Can you work these out from the model? Positions are in its coordinate system, mm. A direction names the side the tool comes from. Round coordinates to 2 decimals unless told otherwise and drop trailing zeros. Loops run counter-clockwise (first coordinate to the right, second up) from the corner with the lowest first, then second, coordinate; pieces in that order, holes last.
```python
from build123d import *

# Parameters (mm, degrees)
BOSS_EXTRUDE1_DEPTH = 9.525
SKETCH2_R           = 1.905
CUT_EXTRUDE1_DEPTH  = 9.525
SKETCH3_R           = 2.286
CUT_EXTRUDE2_DEPTH  = 78.455641076


with BuildPart() as part:
    # Sketch1 → Boss-Extrude1 (new body)
    with BuildSketch(Plane(origin=(0, 0, 0), x_dir=(0, 0, -1), z_dir=(1, 0, 0))):
        Polygon((0, 0), (-25.4, 0), (25.4, 72.549918742), (25.4, 12.7), (0, 12.7), align=None)
    extrude(amount=BOSS_EXTRUDE1_DEPTH)

    # Sketch2 → Cut-Extrude1 (cut)
    with BuildSketch(Plane.XZ.offset(-12.7)):
        with Locations(Location((4.7625, -19.05, 0), (0, 0, 270))):
            Circle(SKETCH2_R)
        with Locations(Location((4.7625, -6.35, 0), (0, 0, 270))):
            Circle(SKETCH2_R)
    extrude(amount=-CUT_EXTRUDE1_DEPTH, mode=Mode.SUBTRACT)

    # Sketch3 → Cut-Extrude2 (cut, through all)
    with BuildSketch(Plane(origin=(9.525, 0, 0), x_dir=(0, 0, -1), z_dir=(1, 0, 0))):
        with Locations((-6.35, 16.135332376)):
            Circle(SKETCH3_R)
        with Locations((15.503262225, 47.345025264)):
            Circle(SKETCH3_R)
    extrude(amount=-CUT_EXTRUDE2_DEPTH, mode=Mode.SUBTRACT)


solid = part.part
```
(1) Which directions (+Z, -Z, +X, -X, +Y, -Y) give clear straight access to the entire face, cutting with the end or side of a thin tool? Please do faces 4 (the flat face through (5, 22.225, -6)), 5 (the flat face through (9.525, 26, -10)), 6 (the flat face through (5, 12.7, -13)).
(2) We'd pull the mould along Z, two halves only. Please class faces 1 (the flat face through (5, 43, -25.4)), 2 (the cylindrical face through (3.6, 17.4, -4.84)), 3 (the flat face through (0, 26, -10)): released by +Z, released by -Z, zero draft, split by the parting line, or undercut.
(3) If I drill on line 1 (Z direction, x = 5.5, y = 15); line 2 (Z direction, x = 5.5, y = 17.5); line 3 (X direction, y = 16, z = -19) (3 decimals), over which ranges is the centre line in solid material (lowest first)?
(4) Suppose I cut it at D-D (y = 54.5). Write out the boundary of the cut face in (x, z) (3 decimals), then the cut area to 3 significant figures.
(5) Suppose I cut it at B-B (z = 6.35). Write out the boundary of the cut face in (x, y) (3 decimals), then the cut area to 3 significant figures.
(6) For pin 1 (1.9 mm diameter, centred on x = 4.5, z = -19, fed in from -Y) (3 decimals); pin 2 (5 mm diameter, centred on x = 5.5, z = -12.5, fed in from -Y); pin 3 (3.5 mm diameter, centred on x = 4.76, z = -19.05, fed in from +Y), each with a flat end and sliding along its axis, tell me the tip position at first contact or that it passes through.
(7) Suppose I cut it at C-C (z = -6.35). Write out the boundary of the cut face in (x, y) (1 decimal), then the cut area to 3 significant figures.
(8) Suppose I cut it at A-A (x = 8.5). Write out the boundary of the cut face in (y, z).
Check result:
1. face 4: -Y
1. face 5: +Z, -Z, +X, +Y, -Y
1. face 6: -Z, +X, -X, -Y
2. face 1: released by -Z
2. face 2: undercut
2. face 3: zero draft
3. line 1: z = -25.4 to -20.81, -17.29 to -8.11, -4.59 to 4.37, 8.33 to 14.9
3. line 2: z = -25.4 to -20.81, -17.29 to -8.11, -4.59 to 4.52, 8.18 to 13.15
3. line 3: x = 0 to 2.858, 6.667 to 9.525
4. outline: (0, -25.4) - (9.525, -25.4) - (9.525, -12.761) - (0, -12.761) - close
4. area: 120 mm2
5. outline: (0, 0) - (9.525, 0) - (9.525, 13.849) - (0, 13.849) - close; (0, 18.421) - (9.525, 18.421) - (9.525, 27.206) - (0, 27.206) - close
5. area: 216 mm2
6. pin 1: stops at y = 22.225
6. pin 2: stops at y = 12.7
6. pin 3: stops at y = 65.98
7. outline: (0, 12.7) - (2.9, 12.7) - (2.9, 22.2) - (6.7, 22.2) - (6.7, 12.7) - (9.5, 12.7) - (9.5, 45.3) - (0, 45.3) - close
7. area: 275 mm2
8. outline: (0, 0) - (12.7, 0) - (12.7, -25.4) - (72.55, -25.4) - (0, 25.4) - close; hole circle Ø4.57 at (16.14, 6.35); hole circle Ø4.57 at (47.35, -15.5)
